Model file for the job. Use its own axes, mm. A direction names the side the tool comes from. Coordinates: 2 decimals unless noted, no trailing zeros. Write each loop counter-clockwise with the first axis right and the second up, starting at its lowest first coordinate (ties: lowest second). Pieces come first, ordered by that corner, then holes. Notation, with made-up numbers: (23.25, -26.5) - (48.25, -26.5) arc R27 ccw to (48.25, -0.5) - close; hole circle Ø4 at (-31, -21). An arc over 180 degrees is marked (long way). Put each result on its own line as item: value. Start each with the question number.
1. Saw through at A-A, the plane y = 3.75. Write the cut outline in (x, z) (3 decimals), plus the area to 3 significant figures.
2. Saw through at C-C, the plane z = -6. Write the cut outline in (x, y).
3. Saw through at D-D, the plane x = 0. Write the cut outline in (y, z) (3 decimals), plus the area to 3 significant figures.
4. Saw through at B-B, the plane x = 12.5. Write the cut outline in (y, z).
5. Drop flat-ended pins along their axis: P1, Ø1.5, axis at x = -0.5, z = 7.5, coming from the -Y side; P2, Ø2, axis at x = -7, y = 1.5, coming from the +Z side; P3, Ø2, axis at x = 8, y = 3, coming from the +Z side. Give the stop position or say it passes through.
6. Drill centre lines: L1, parallel to X at y = 2, z = -12; L2, parallel to Z at x = 13.5, y = 4; L3, parallel to Z at x = 2, y = 2. Where is each one in solid material? Low to high. Write a range as from..to.
7. Which spindle directions (+Z, -Z, +X, -X, +Y, -Y) get a long thin tool onto all of the face, cutting with end or side? Do faces 1 (the face through (0, 6.35, -8)), 2 (the face through (-2.4, 2.46, 10.81)). Say none if no direction does.
8. Pull direction X, two halves, no side cores. Call faces 3 (the face through (15.85, 3.13, -15.93)), 4 (the face through (-16.09, 3.13, -4)), 5 (the face through (12.09, 3.13, 14.1)), 6 (the face through (-0.2, 5, 7.2)): released by +X, released by -X, zero draft, split by the parting line, or undercut.
```python
from build123d import *

# Parameters (mm, degrees)
SKETCH1_R             = 7
BOSS_EXTRUDE1_DEPTH   = 6.35
SKETCH1_3_R           = 11.075
CUT_EXTRUDE1_DEPTH    = 5
M5X0_8_TAPPED_HOLE1_D = 4.2


with BuildPart() as part:
    # Sketch1 → Boss-Extrude1 (new body)
    with BuildSketch(Plane(origin=(0, 0, 0), x_dir=(1, 0, 0), z_dir=(0, 1, 0))):
        with BuildLine():
            Line((-12, 17.5), (12, 17.5))
            ThreePointArc((12, 17.5), (15.889087297, 15.889087297), (17.5, 12))
            Line((17.5, 12), (17.5, -12))
            ThreePointArc((17.5, -12), (15.511287903, -16.233303351), (10.983324632, -17.405217035))
            Line((10.983324632, -17.405217035), (-2.78661476, -14.81520851))
            ThreePointArc((-2.78661476, -14.81520851), (-10.659634726, -10.659634726), (-14.81520851, -2.78661476))
            Line((-14.81520851, -2.78661476), (-17.405217035, 10.983324632))
            ThreePointArc((-17.405217035, 10.983324632), (-16.233303351, 15.511287903), (-12, 17.5))
        make_face()
        Circle(SKETCH1_R, mode=Mode.SUBTRACT)
    extrude(amount=BOSS_EXTRUDE1_DEPTH)

    # Sketch1<3> → Cut-Extrude1 (cut)
    with BuildSketch(Plane(origin=(0, 0, 0), x_dir=(1, 0, 0), z_dir=(0, 1, 0))):
        Circle(SKETCH1_3_R)
    extrude(amount=CUT_EXTRUDE1_DEPTH, mode=Mode.SUBTRACT)

    # M5x0.8 Tapped Hole1 (through all)
    with Locations(Plane(origin=(12, 6.35, -12), x_dir=(0, 0, 1), z_dir=(0, 1, 0))):
        with Locations((0, 0), (24, 0), (0, -24)):
            Hole(M5X0_8_TAPPED_HOLE1_D / 2)


solid = part.part
```
Final values:
1. outline: (-17.405, -10.983) arc R5.5 ccw to (-12, -17.5) - (12, -17.5) arc R5.5 ccw to (17.5, -12) - (17.5, 12) arc R5.5 ccw to (10.983, 17.405) - (-2.787, 14.815) arc R15.075 ccw to (-14.815, 2.787) - close; hole circle Ø4.2 at (-12, -12); hole circle Ø22.15 at (0, 0); hole circle Ø4.2 at (12, -12); hole circle Ø4.2 at (12, 12)
1. area: 627 mm²
2. outline: (-16.47, 0) - (-9.31, 0) - (-9.31, 5) - (-3.61, 5) - (-3.61, 6.35) - (-16.47, 6.35) - close; (3.61, 5) - (9.31, 5) - (9.31, 0) - (17.5, 0) - (17.5, 6.35) - (3.61, 6.35) - close
3. outline: (0, -17.5) - (6.35, -17.5) - (6.35, -7) - (5, -7) - (5, -11.075) - (0, -11.075) - close; (0, 11.075) - (5, 11.075) - (5, 7) - (6.35, 7) - (6.35, 15.339) - (0, 15.339) - close
3. area: 78.9 mm²
4. outline: (0, -17.48) - (6.35, -17.48) - (6.35, -14.04) - (0, -14.04) - close; (0, -9.96) - (6.35, -9.96) - (6.35, 9.96) - (0, 9.96) - close; (0, 14.04) - (6.35, 14.04) - (6.35, 17.48) - (0, 17.48) - close
5. P1: stops at y = 5
5. P2: stops at z = 13.83
5. P3: stops at z = 17.03
6. L1: x = -17.5..-14.1, -9.9..9.9, 14.1..17.5
6. L2: z = -17.29..-13.47, -10.53..10.53, 13.47..17.29
6. L3: z = -17.5..-10.89, 10.89..15.72
7. face 1: +Z, -Z, +X, -X, +Y
7. face 2: -Y
8. face 3: released by +X
8. face 4: released by -X
8. face 5: undercut
8. face 6: undercut
